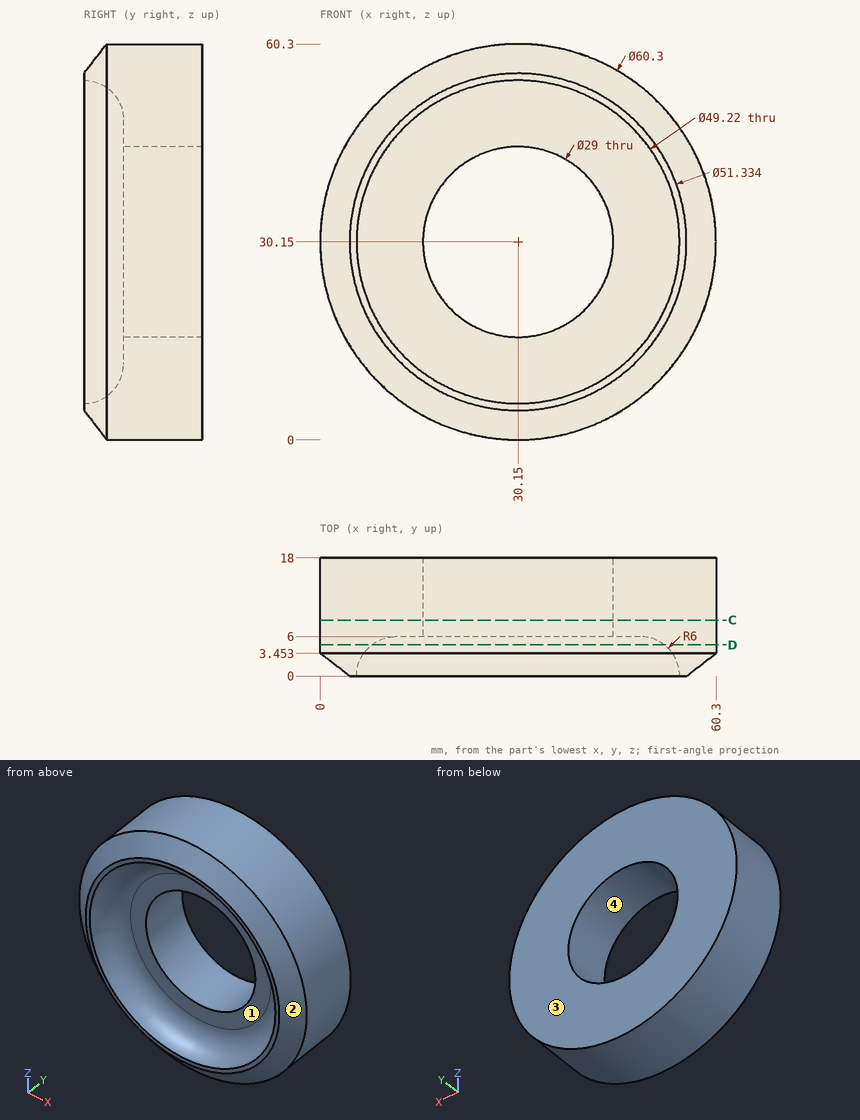
Check sheet for the drawn part. Datum: minimum x, y, z corner. Units: mm. Give positions to 0.01 mm unless a question says otherwise; leave off trailing zeros. Order: outer loops, then holes, each group sorted by start corner. A loop starts at its lowest first (then second) coordinate and runs counter-clockwise, first axis right, second up. Notation, with made-up numbers: (-37.5, 20) -> (-18.5, 20) arc R17 cw to (-18.5, 41) -> close; hole circle Ø2 at (28.25, 81.25). An arc over 180 degrees is marked (long way). Use a Markdown table: item, result.
1) Section check C-C, the plane y = 8.5. Record the boundary of the cut face in (x, z).
Results:
| item | result |
|---|---|
| outline | circle Ø60.3 at (30.15, 30.15); hole circle Ø29 at (30.15, 30.15) |
2) Section check D-D, the plane y = 4.75. Record the boundary of the cut face in (x, z).
Results:
| item | result |
|---|---|
| outline | circle Ø60.3 at (30.15, 30.15); hole circle Ø44.55 at (30.15, 30.15) |
3) Depth check by flat-ended pin: pin 1 Ø23 at (x, z) = (30.15, 30.15) entering from -Y; pin 2 Ø8 at (x, y) = (16.5, 15) entering from +Z; pin 3 Ø8 at (x, y) = (12.5, 5.5) entering from +Z; pin 4 Ø8 at (x, z) = (45, 24.5) entering from -Y. Enter the tip coordinate at first touch or a pass-through.
Results:
| item | result |
|---|---|
| pin 1 | through |
| pin 2 | z = 58.71 |
| pin 3 | z = 57.03 |
| pin 4 | y = 5.86 |
4) Mould release check, pull along X, two halves, no side actions. Record for the marked faces 1, 2, 3 and 4: pulls with the +X half, pulls with the -X half, needs draft (parallel to the pull), parting line crosses it, or undercut.
Results:
| item | result |
|---|---|
| face 1 | undercut |
| face 2 | parting line crosses it |
| face 3 | needs draft |
| face 4 | undercut |
5) Material ranges on probe 1 along Y at (x, z) = (41, 15); probe 2 along X at (y, z) = (2, 26.5) (1 decimal); probe 3 along X at (y, z) = (16.5, 21), recorded low to high.
Results:
| item | result |
|---|---|
| probe 1 | 6 to 18 |
| probe 2 | 2.1 to 6.2, 54.1 to 58.2 |
| probe 3 | 1.42 to 18.9, 41.4 to 58.88 |
